Verification items for this drawing (mm, ordinates from the low corner). A direction names the side the tool comes from. Round coordinates to 2 decimals unless told otherwise and drop trailing zeros. Write each loop counter-clockwise with the first axis right and the second up, starting at its lowest first coordinate (ties: lowest second). Pieces come first, ordered by that corner, then holes. Notation, with made-up numbers: (44.5, 56.5) -> (54.5, 56.5) arc R24 ccw to (54.5, 80.5) -> close; hole circle Ø10 at (66, 37). An arc over 180 degrees is marked (long way). Use one line per item in the form item = value. Start each with the question number.
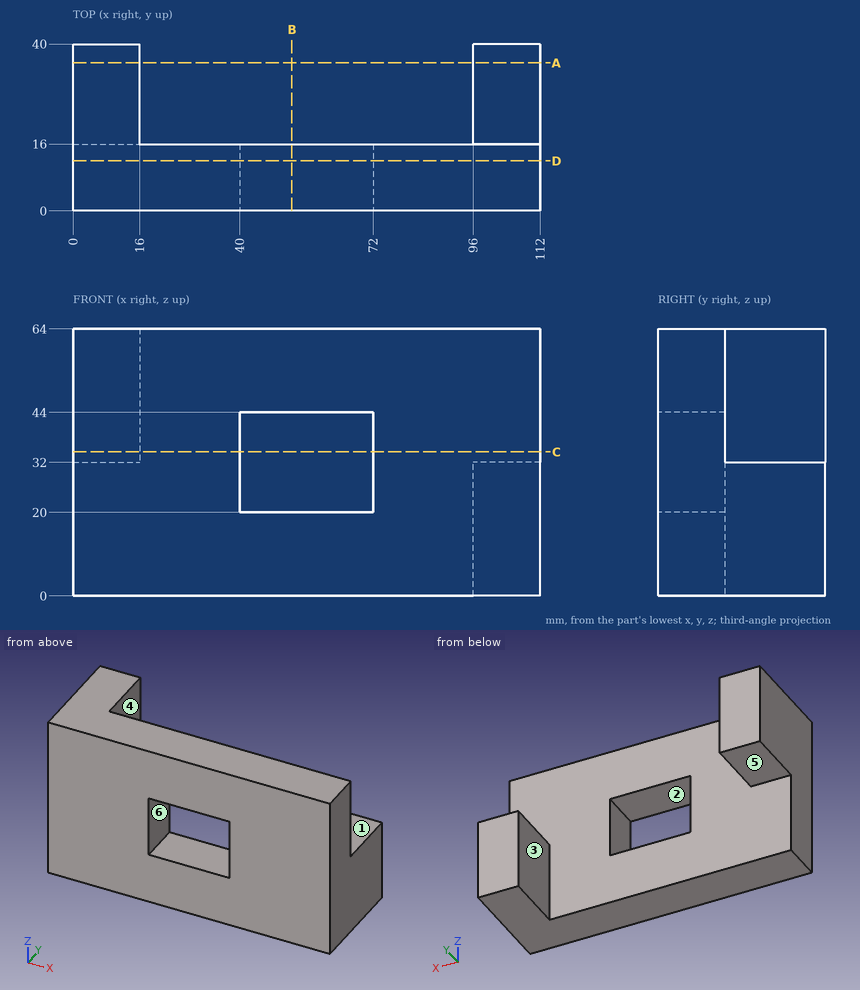
1. Sectioned sample at C-C (z = 34.5). Enter the section's corners in (x, y).
2. Sectioned sample at B-B (x = 52.5). Enter the section's corners in (y, z), and give its area (3 significant figures).
3. Scan lines: probe 1 along X at (y, z) = (2.5, 39); probe 2 along Z at (x, y) = (42.5, 4); probe 3 along X at (y, z) = (21, 8). Record each from-to range of solid material in increasing order.
4. Mould release check, pull along Z, two halves, no side actions. Record for the marked faces 1, 2 and 3: +Z half, -Z half, draft (parallel to the pull), parting line (faces both ways), or undercut.
5. Depth check by flat-ended pin: pin 1 (5 mm diameter, centred on x = 74.5, y = 9.5, fed in from -Z); pin 2 (8 mm diameter, centred on x = 31.5, z = 10, fed in from +Y); pin 3 (19 mm diameter, centred on y = 33, z = 17, fed in from -X); pin 4 (17.5 mm diameter, centred on x = 5.5, y = 33, fed in from -Z). Enter the tip coordinate at first touch or a pass-through.
6. Sectioned sample at A-A (y = 35.5). Enter the section's corners in (x, z), and give its area (3 significant figures).
7. Sectioned sample at D-D (y = 12). Enter the section's corners in (x, z), and give its area (3 significant figures).
8. Tool access check on the marked faces 4, 5 and 6. Record the directions out of +Z, -Z, +X, -X, +Y, -Y that give a thin tool (end or side, any length) a straight path to the whole face; none if there is none.
Returned:
q1.outline = (0, 0) -> (40, 0) -> (40, 16) -> (16, 16) -> (16, 40) -> (0, 40) -> close; (72, 0) -> (112, 0) -> (112, 16) -> (72, 16) -> close
q2.outline = (0, 0) -> (16, 0) -> (16, 20) -> (0, 20) -> close; (0, 44) -> (16, 44) -> (16, 64) -> (0, 64) -> close
q2.area = 640 mm^2
q3.probe_1 = 0 to 40, 72 to 112
q3.probe_2 = 0 to 20, 44 to 64
q3.probe_3 = 96 to 112
q4.face_1 = +Z half
q4.face_2 = undercut
q4.face_3 = draft
q5.pin_1 = 0
q5.pin_2 = 16
q5.pin_3 = 96
q5.pin_4 = 32
q6.outline = (0, 32) -> (16, 32) -> (16, 64) -> (0, 64) -> close; (96, 0) -> (112, 0) -> (112, 32) -> (96, 32) -> close
q6.area = 1,020 mm^2
q7.outline = (0, 0) -> (112, 0) -> (112, 64) -> (0, 64) -> close; hole (40, 20) -> (72, 20) -> (72, 44) -> (40, 44) -> close
q7.area = 6,400 mm^2
q8.face_4 = +Z, -Z, +X, +Y
q8.face_5 = -Z, -X, +Y
q8.face_6 = +Y, -Y
